```python
from build123d import *

# Parameters (mm, degrees)
F0_W     = 3
F0_H     = 7
F1_DEPTH = 7
F2_R     = 3
F3_R     = 1.6
F4_DEPTH = 25
F5_R     = 1.6
F6_DEPTH = 25


with BuildPart() as f1:
    # F0 (on Top) → F1 (new body)
    with BuildSketch(Plane.XY):
        with Locations((-18.815929, 24.224132)):
            Rectangle(F0_W, F0_H)
        with BuildLine():
            Line((5.684071, 11.664157), (5.684071, -16.215892))
            ThreePointArc((5.684071, -16.215892), (5.228779, -19.377972), (3.884071, -22.275868))
            Line((3.884071, -22.275868), (-20.315929, -22.275868))
            Line((-20.315929, -22.275868), (-20.315929, -25.275868))
            Line((-20.315929, -25.275868), (-17.315929, -25.275868))
            Line((-17.315929, -25.275868), (5.382678, -25.275868))
            ThreePointArc((5.382678, -25.275868), (7.827057, -21.069053), (8.684071, -16.279711))
            Line((8.684071, -16.279711), (8.684071, 11.727975))
            ThreePointArc((8.684071, 11.727975), (7.827057, 16.517318), (5.382678, 20.724132))
            Line((5.382678, 20.724132), (-17.315929, 20.724132))
            Line((-17.315929, 20.724132), (-20.315929, 20.724132))
            Line((-20.315929, 20.724132), (-20.315929, 17.724132))
            Line((-20.315929, 17.724132), (3.884071, 17.724132))
            ThreePointArc((3.884071, 17.724132), (5.228779, 14.826237), (5.684071, 11.664157))
        make_face()
        with Locations((-18.815929, -28.775868)):
            Rectangle(F0_W, F0_H)
    extrude(amount=F1_DEPTH)

    # F2
    f2_edges = [f1.edges().sort_by_distance(p)[0] for p in [
        (-18.815929, 27.724132, 0),
        (-18.815929, 27.724132, 7),
        (-18.815929, -32.275868, 0),
        (-18.815929, -32.275868, 7),
    ]]
    fillet(f2_edges, radius=F2_R)

    # F3 (on face) → F4 (cut)
    with BuildSketch(Plane.YZ.offset(-17.315929)):
        with Locations((-28.775868, 3.5)):
            Circle(F3_R)
    extrude(amount=-F4_DEPTH, mode=Mode.SUBTRACT)

    # F5 (on face) → F6 (cut)
    with BuildSketch(Plane.YZ.offset(-17.315929)):
        with Locations((24.224132, 3.5)):
            Circle(F5_R)
    extrude(amount=-F6_DEPTH, mode=Mode.SUBTRACT)


solid = f1.part
```
Geometry: final body of the model. Coordinates: model frame, mm. A direction names the side the tool comes from. Coordinates: 2 decimals unless noted, no trailing zeros. Order: outer loops, then holes, each group sorted by start corner. A loop starts at its lowest first (then second) coordinate and runs counter-clockwise, first axis right, second up. Notation, with made-up numbers: M 41,20.25 L 93,20.25 A20 ccw 93,45.25 Z; hole C -10,25 d11. An arc over 180 degrees is marked long. Answer in a Markdown table with one row per item. Add a question column.
Q1. Section query A-A on x = -3. Return the cut outline in (y, z), and give its area (3 significant figures).
Q2. Contact query for flat-ended pins moving along their axis: P1, Ø3, axis at x = 2, z = 5.5, coming from the +Y side; P2, Ø2, axis at x = 3, z = 4, coming from the -Y side. Output: stop coordinate, or through.
Q3. Line query: L1, parallel to Y at x = -6.25, z = 5.5; L2, parallel to X at y = 12, z = 3; L3, parallel to X at y = -28, z = 6.5. Output: solid intervals per line, ascending.
Q4. Section query B-B on z = 1.25. Return the cut outline in (x, y).
Q5. Reachability of faces 4 (the flat face through (6, -2, 7)), 5 (the flat face through (-6, 20.724, 3)), 6 (the cylindrical face through (5.216, 14.869, 3.451)), 7 (the cylindrical face through (-18.79, -31.42, 6.1)), 8 (the flat face through (-17.316, -27, 3)) from +Z, -Z, +X, -X, +Y, -Y: full face, straight path, thin tool, end or side. Return the list, or none.
Q6. Mould query, pull axis Y, two halves, no side actions, for faces 1 (the flat face through (-8, -22.276, 3)), 2 (the cylindrical face through (7.85, 16.45, 3.45)), 3 (the flat face through (-20.316, -26, 3)). Classes: released by +Y, released by -Y, zero draft, split by the parting line, or undercut.
Q7. Section query D-D on x = 6.5. Return the cut outline in (y, z), and give its area (3 significant figures).
Q8. Section query C-C on y = -9. Return the cut outline in (x, z).
Completed:
| question | item | result |
|---|---|---|
| 1 | outline | M -25.28,0 L -22.28,0 L -22.28,7 L -25.28,7 Z; M 17.72,0 L 20.72,0 L 20.72,7 L 17.72,7 Z |
| 1 | area | 42.0 mm2 |
| 2 | P1 | stops at y = 20.72 |
| 2 | P2 | stops at y = -25.28 |
| 3 | L1 | y = -25.28 to -22.28, 17.72 to 20.72 |
| 3 | L2 | x = 5.68 to 8.68 |
| 3 | L3 | x = -20.32 to -17.32 |
| 4 | outline | M -20.32,-31.71 L -17.32,-31.71 L -17.32,-25.28 L 5.38,-25.28 A14 ccw 8.68,-16.28 L 8.68,11.73 A14 ccw 5.38,20.72 L -17.32,20.72 L -17.32,27.16 L -20.32,27.16 L -20.32,17.72 L 3.88,17.72 A11 cw 5.68,11.66 L 5.68,-16.22 A11 cw 3.88,-22.28 L -20.32,-22.28 Z |
| 5 | face 4 | +Z, +X, -X, +Y, -Y |
| 5 | face 5 | +Z, -Z, +X, +Y |
| 5 | face 6 | +Z, -Z, -X |
| 5 | face 7 | +Z, +X, -X, -Y |
| 5 | face 8 | +Z, -Z, +X, -Y |
| 6 | face 1 | undercut |
| 6 | face 2 | released by +Y |
| 6 | face 3 | zero draft |
| 7 | outline | M -23.75,0 L 19.2,0 L 19.2,7 L -23.75,7 Z |
| 7 | area | 301 mm2 |
| 8 | outline | M 5.68,0 L 8.68,0 L 8.68,7 L 5.68,7 Z |
